from build123d import *

# Parameters (mm, degrees)
ROTOR_SKETCH_R = 2.5
ROTOR_DEPTH    = 14


with BuildPart() as part:
    # Rotor_Sketch → Rotor (new body)
    with BuildSketch(Plane.XY):
        with BuildLine():
            Line((-8.75, 33.737818734), (-8.75, 23.418742494))
            ThreePointArc((-8.75, 23.418742494), (-17.67766953, 17.67766953), (-23.418742494, 8.75))
            Line((-23.418742494, 8.75), (-33.737818734, 8.75))
            ThreePointArc((-33.737818734, 8.75), (-34.854022909, 0), (-33.737818734, -8.75))
            Line((-33.737818734, -8.75), (-23.418742494, -8.75))
            ThreePointArc((-23.418742494, -8.75), (-17.67766953, -17.67766953), (-8.75, -23.418742494))
            Line((-8.75, -23.418742494), (-8.75, -33.737818734))
            ThreePointArc((-8.75, -33.737818734), (0, -34.854022909), (8.75, -33.737818734))
            Line((8.75, -33.737818734), (8.75, -23.418742494))
            ThreePointArc((8.75, -23.418742494), (17.67766953, -17.67766953), (23.418742494, -8.75))
            Line((23.418742494, -8.75), (33.737818734, -8.75))
            ThreePointArc((33.737818734, -8.75), (34.854022909, 0), (33.737818734, 8.75))
            Line((33.737818734, 8.75), (23.418742494, 8.75))
            ThreePointArc((23.418742494, 8.75), (17.67766953, 17.67766953), (8.75, 23.418742494))
            Line((8.75, 23.418742494), (8.75, 33.737818734))
            ThreePointArc((8.75, 33.737818734), (0, 34.854022909), (-8.75, 33.737818734))
        make_face()
        Circle(ROTOR_SKETCH_R, mode=Mode.SUBTRACT)
    extrude(amount=ROTOR_DEPTH)


solid = part.part
Geometry: final body of the model. Coordinates: model frame, mm. A direction names the side the tool comes from. Round coordinates to 2 decimals unless told otherwise and drop trailing zeros. Loops run counter-clockwise (first coordinate to the right, second up) from the corner with the lowest first, then second, coordinate; pieces in that order, holes last.
Q1. Section B-B on z = 6.5. Return loops of the section in (x, y).
Q2. Pull-direction query (Y, two-part tool) for faces 6 (the cylindrical face through (34.854, -0.124, 6.902)), 7 (the cylindrical face through (0.124, 34.854, 6.902)), 8 (the flat face through (-29, -8.75, 7)), 9 (the cylindrical face through (-0.54, -2.44, 6.9)); classes: released by +Y, released by -Y, zero draft, split by the parting line, or undercut.
Q3. Pin query (flat end, axial travel): P1, Ø5, axis at y = 30, z = 5, coming from the -X side; P2, Ø5, axis at x = -9, z = 12, coming from the +Y side; P3, Ø4, axis at x = -13, z = 3, coming from the +Y side; P4, Ø6, axis at x = 0, y = 0, coming from the -Z side. Return the tip coordinate at first contact, or that it passes through.
Q4. Section D-D on x = 30.5. Return loops of the section in (y, z), plus the area to 3 significant figures.
Q5. Access query for faces 1 (the flat face through (0, 8, 14)), 2 (the flat face through (29, 8.75, 7)), 3 (the flat face through (29, -8.75, 7)), 4 (the flat face through (-29, 8.75, 7)), 5 (the flat face through (-8.75, -29, 7)). Directions: +Z, -Z, +X, -X, +Y, -Y. A direction counts if a zero-diameter tool reaches every point of the face in a straight line with its end or side. Return the directions, or none.
Q6. Section A-A on y = 0. Return loops of the section in (x, z), plus the area to 3 significant figures.
Q7. Material intervals for L1, parallel to Y at x = 0, z = 5; L2, parallel to X at y = 31.5, z = 4.5, sorted ascending.
Evaluation:
1. outline: (-33.74, -8.75) - (-23.42, -8.75) arc R25 ccw to (-8.75, -23.42) - (-8.75, -33.74) arc R34.85 ccw to (8.75, -33.74) - (8.75, -23.42) arc R25 ccw to (23.42, -8.75) - (33.74, -8.75) arc R34.85 ccw to (33.74, 8.75) - (23.42, 8.75) arc R25 ccw to (8.75, 23.42) - (8.75, 33.74) arc R34.85 ccw to (-8.75, 33.74) - (-8.75, 23.42) arc R25 ccw to (-23.42, 8.75) - (-33.74, 8.75) arc R34.85 ccw to start; hole circle Ø5 at (0, 0)
2. face 6: split by the parting line
2. face 7: released by +Y
2. face 8: released by -Y
2. face 9: undercut
3. P1: stops at x = -8.75
3. P2: stops at y = 34.24
3. P3: stops at y = 22.45
3. P4: stops at z = 0
4. outline: (-8.75, 0) - (8.75, 0) - (8.75, 14) - (-8.75, 14) - close
4. area: 245 mm2
5. face 1: +Z, +X, -X, +Y, -Y
5. face 2: +Z, -Z, +X, +Y
5. face 3: +Z, -Z, +X, -Y
5. face 4: +Z, -Z, -X, +Y
5. face 5: +Z, -Z, -X, -Y
6. outline: (-34.85, 0) - (-2.5, 0) - (-2.5, 14) - (-34.85, 14) - close; (2.5, 0) - (34.85, 0) - (34.85, 14) - (2.5, 14) - close
6. area: 906 mm2
7. L1: y = -34.85 to -2.5, 2.5 to 34.85
7. L2: x = -8.75 to 8.75
